from build123d import *

# Parameters (mm, degrees)
ESQUISSE1_R      = 2.5
EXTRUSION1_DEPTH = 3
CONG_1_R         = 15
EXTRUSION2_REACH = 5
ESQUISSE2_W      = 3
ESQUISSE2_H      = 93
ESQUISSE2_W_2    = 300
ESQUISSE2_H_2    = 3


with BuildPart() as part:
    # Esquisse1 → Extrusion1 (new body)
    with BuildSketch(Plane(origin=(0, 0, 0), x_dir=(1, 0, 0), z_dir=(0, 1, 0))):
        Polygon((0, 0), (30, 0), (30, 20), (80, 20), (80, 35), (250, 35), (250, 20), (300, 20), (300, 0), (330, 0), (330, 123), (0, 123), align=None)
        with Locations((10, 113)):
            Circle(ESQUISSE1_R, mode=Mode.SUBTRACT)
        with Locations((320, 113)):
            Circle(ESQUISSE1_R, mode=Mode.SUBTRACT)
        with Locations((10, 12)):
            Circle(ESQUISSE1_R, mode=Mode.SUBTRACT)
        with Locations((320, 12)):
            Circle(ESQUISSE1_R, mode=Mode.SUBTRACT)
        with BuildLine():
            Line((300, 93), (300, 55))
            ThreePointArc((300, 55), (290, 45), (280, 55))
            Line((280, 55), (280, 93))
            ThreePointArc((280, 93), (290, 103), (300, 93))
        make_face(mode=Mode.SUBTRACT)
        with BuildLine():
            Line((30, 93), (30, 55))
            ThreePointArc((30, 55), (40, 45), (50, 55))
            Line((50, 55), (50, 93))
            ThreePointArc((50, 93), (40, 103), (30, 93))
        make_face(mode=Mode.SUBTRACT)
    extrude(amount=EXTRUSION1_DEPTH)

    # Congé1
    cong_1_edges = [part.edges().sort_by_distance(p)[0] for p in [
        (0, 1.5, -123),
        (330, 1.5, -123),
        (330, 1.5, 0),
        (0, 1.5, 0),
    ]]
    fillet(cong_1_edges, radius=CONG_1_R)

    # Esquisse2 → Extrusion2 (cut, up to next)
    with BuildSketch(Plane(origin=(0, 3, 0), x_dir=(1, 0, 0), z_dir=(0, 1, 0)), mode=Mode.PRIVATE) as extrusion2_sk1:
        with Locations((1.5, 61.5)):
            Rectangle(ESQUISSE2_W, ESQUISSE2_H)
    extrusion2_tool1 = extrude(extrusion2_sk1.sketch, amount=-EXTRUSION2_REACH, mode=Mode.PRIVATE) & part.part
    add(extrusion2_tool1.solids().sort_by_distance((1.5, 3, -61.5))[0], mode=Mode.SUBTRACT)
    # Esquisse2 → Extrusion2 (cut, up to next)
    with BuildSketch(Plane(origin=(0, 3, 0), x_dir=(1, 0, 0), z_dir=(0, 1, 0)), mode=Mode.PRIVATE) as extrusion2_sk2:
        with Locations((165, 121.5)):
            Rectangle(ESQUISSE2_W_2, ESQUISSE2_H_2)
    extrusion2_tool2 = extrude(extrusion2_sk2.sketch, amount=-EXTRUSION2_REACH, mode=Mode.PRIVATE) & part.part
    add(extrusion2_tool2.solids().sort_by_distance((165, 3, -121.5))[0], mode=Mode.SUBTRACT)
    # Esquisse2 → Extrusion2 (cut, up to next)
    with BuildSketch(Plane(origin=(0, 3, 0), x_dir=(1, 0, 0), z_dir=(0, 1, 0)), mode=Mode.PRIVATE) as extrusion2_sk3:
        with Locations((328.5, 61.5)):
            Rectangle(ESQUISSE2_W, ESQUISSE2_H)
    extrusion2_tool3 = extrude(extrusion2_sk3.sketch, amount=-EXTRUSION2_REACH, mode=Mode.PRIVATE) & part.part
    add(extrusion2_tool3.solids().sort_by_distance((328.5, 3, -61.5))[0], mode=Mode.SUBTRACT)


solid = part.part
Geometry: final body of the model. Coordinates: model frame, mm. A direction names the side the tool comes from. Give positions to 0.01 mm unless a question says otherwise; leave off trailing zeros. Write each loop counter-clockwise with the first axis right and the second up, starting at its lowest first coordinate (ties: lowest second). Pieces come first, ordered by that corner, then holes. Notation, with made-up numbers: (-11, -7) -> (12, -7) arc R22 ccw to (12, 23) -> close; hole circle Ø5 at (19.5, 35). An arc over 180 degrees is marked (long way). Answer in a Markdown table with one row per item.
(1) Section query D-D on z = -23. Return loops of the section in (x, y).
Answers below:
| item | result |
|---|---|
| outline | (3, 0) -> (80, 0) -> (80, 3) -> (3, 3) -> close; (250, 0) -> (327, 0) -> (327, 3) -> (250, 3) -> close |
(2) Section query B-B on z = -65. Return loops of the section in (x, y).
Answers below:
| item | result |
|---|---|
| outline | (3, 0) -> (30, 0) -> (30, 3) -> (3, 3) -> close; (50, 0) -> (280, 0) -> (280, 3) -> (50, 3) -> close; (300, 0) -> (327, 0) -> (327, 3) -> (300, 3) -> close |
(3) Draft query along X for faces 3 (the cylindrical face through (290, 1, -103)), 4 (the cylindrical face through (40, 1, -103)), 5 (the cylindrical face through (325.49, 1.52, -118.72)), 6 (the flat face through (163, 0, -76)). Return one class per face: +X half, -X half, draft (parallel to the pull), parting line (faces both ways), or undercut.
Answers below:
| item | result |
|---|---|
| face 3 | undercut |
| face 4 | undercut |
| face 5 | +X half |
| face 6 | draft |
(4) Set-up query: faces 1 (the cylindrical face through (290, 1, -45)), 2 (the cylindrical face through (4.51, 1.52, -4.28)). Return all of +Z, -Z, +X, -X, +Y, -Y with unobstructed straight access to the full face (end or side cutting, diameter ignored); none if empty.
Answers below:
| item | result |
|---|---|
| face 1 | +Y, -Y |
| face 2 | +Z, -X, +Y, -Y |
(5) Ray query, line 1 along X through (y, z) = (2, -60); line 2 along X through (y, z) = (2.75, -47); line 3 along X through (y, z) = (1.75, -12). Return the intervals inside material, ascending. Write a range as [from, to].
Answers below:
| item | result |
|---|---|
| line 1 | [3, 30], [50, 280], [300, 327] |
| line 2 | [3, 34], [46, 284], [296, 327] |
| line 3 | [0.3, 7.5], [12.5, 30], [300, 317.5], [322.5, 329.7] |
(6) Pin query (flat end, axial travel): pin 1 (1.5 mm diameter, centred on x = 118, y = 2, fed in from -Z); pin 2 (4.5 mm diameter, centred on x = 320, z = -12, fed in from +Y); pin 3 (1.5 mm diameter, centred on x = 328.5, y = 2, fed in from -Z); pin 4 (0.9 mm diameter, centred on x = 192.5, y = 1.5, fed in from +Z). Return the tip coordinate at first contact, or that it passes through.
Answers below:
| item | result |
|---|---|
| pin 1 | z = -120 |
| pin 2 | through |
| pin 3 | z = -115.9 |
| pin 4 | z = -35 |
(7) Section query A-A on y = 0.45. State how many separate pieces and enclosed holes the cut face has, then the cut area to 3 significant figures.
Answers below:
| item | result |
|---|---|
| separate pieces | 1 |
| enclosed holes | 6 |
| area | 28,800 mm^2 |
(8) Section query C-C on x = 290. Return loops of the section in (y, z), then the cut area to 3 significant figures.
Answers below:
| item | result |
|---|---|
| outline | (0, -120) -> (3, -120) -> (3, -103) -> (0, -103) -> close; (0, -45) -> (3, -45) -> (3, -20) -> (0, -20) -> close |
| area | 126 mm^2 |
